```python
from build123d import *

# Parameters (mm, degrees)
CROQUIS1_R                 = 35
SALIENTE_EXTRUIR1_DEPTH    = 14
CROQUIS2_R                 = 17.5
CORTAR_EXTRUIR1_DEPTH      = 52.439284598
VACIADO1_T                 = -2
CHAFL_N1_SIZE              = 0.5
CHAFL_N1_SIZE2             = 1.866025404
CROQUIS5_R                 = 2.5
SALIENTE_EXTRUIR2_DEPTH    = 14
REDONDEO2_R                = 4
CORTAR_EXTRUIR2_DEPTH      = 51.931326337
CORTAR_EXTRUIR2_DEPTH_BACK = 51.931326337
CORTAR_EXTRUIR3_DEPTH      = 51.931326474
CORTAR_EXTRUIR3_DEPTH_BACK = 51.931326474


with BuildPart() as part:
    # Croquis1 → Saliente-Extruir1 (new body)
    with BuildSketch(Plane.XY):
        Circle(CROQUIS1_R)
    extrude(amount=SALIENTE_EXTRUIR1_DEPTH)

    # Croquis2 → Cortar-Extruir1 (cut, through all)
    with BuildSketch(Plane.XY.offset(14)):
        Circle(CROQUIS2_R)
    extrude(amount=-CORTAR_EXTRUIR1_DEPTH, mode=Mode.SUBTRACT)

    # Vaciado1
    vaciado1_openings = [part.faces().sort_by_distance(p)[0] for p in [
        (-34.010050506, 0, 14),
    ]]
    offset(amount=VACIADO1_T, openings=vaciado1_openings, kind=Kind.INTERSECTION)

    # Chaflán1
    chafl_n1_edges = [part.edges().sort_by_distance(p)[0] for p in [
        (-17.5, 0, 14),
    ]]
    chafl_n1_side = [part.faces().sort_by_distance(p)[0] for p in [
        (-18.948456711, 0, 14),
    ]]
    chamfer(chafl_n1_edges, length=CHAFL_N1_SIZE, length2=CHAFL_N1_SIZE2, reference=chafl_n1_side[0])

    # Croquis5 → Saliente-Extruir2 (add, through all)
    with BuildSketch(Plane(origin=(0, 0, 0), x_dir=(-1, 0, 0), z_dir=(0, 0, -1))):
        with Locations((0, 17.5)):
            Circle(CROQUIS5_R)
    extrude(amount=-SALIENTE_EXTRUIR2_DEPTH)

    # Redondeo1: read off the stored shape, not the designer's step
    # Redondeo1 outline → Redondeo1 (revolve)
    with BuildSketch(Plane.XZ):
        with BuildLine():
            ThreePointArc((21.5, 2), (20.085786438, 2.585786438), (19.5, 4))
            Line((19.5, 4), (19.5, 2))
            Line((19.5, 2), (21.5, 2))
        make_face()
        with BuildLine():
            ThreePointArc((33, 4), (32.414213562, 2.585786438), (31, 2))
            Line((31, 2), (33, 2))
            Line((33, 2), (33, 4))
        make_face()
    revolve(axis=Axis((0, 0, 0), (0, 0, 1)))

    # Redondeo2
    redondeo2_edges = [part.edges().sort_by_distance(p)[0] for p in [
        (-35, 0, 0),
    ]]
    fillet(redondeo2_edges, radius=REDONDEO2_R)

    # Croquis3 → Cortar-Extruir2 (cut, two sides: drawn at the far end of the back side and taken through both)
    with BuildSketch(Plane.XY.offset(2).offset(-CORTAR_EXTRUIR2_DEPTH_BACK)):
        with BuildLine():
            Line((8.410016673, 26.432172655), (2.046055643, 20.068211625))
            ThreePointArc((2.046055643, 20.068211625), (-2.196585045, 20.068211625), (-2.196585045, 24.310852312))
            Line((-2.196585045, 24.310852312), (4.167375986, 30.674813342))
            ThreePointArc((4.167375986, 30.674813342), (8.410016673, 30.674813342), (8.410016673, 26.432172655))
        make_face()
    extrude(amount=CORTAR_EXTRUIR2_DEPTH + CORTAR_EXTRUIR2_DEPTH_BACK, mode=Mode.SUBTRACT)

    # Croquis4 → Cortar-Extruir3 (cut, two sides: drawn at the far end of the back side and taken through both)
    with BuildSketch(Plane.XY.offset(2).offset(-CORTAR_EXTRUIR3_DEPTH_BACK)):
        Polygon((5.089600939, 21.651424089), (4.627973548, 20.226390042), (6.318861503, 19.678641589), (6.081885084, 18.947100367), (7.993733444, 19.923368498), (7.017465313, 21.835216858), (6.780488894, 21.103675636), align=None)
    extrude(amount=CORTAR_EXTRUIR3_DEPTH + CORTAR_EXTRUIR3_DEPTH_BACK, mode=Mode.SUBTRACT)


solid = part.part
```
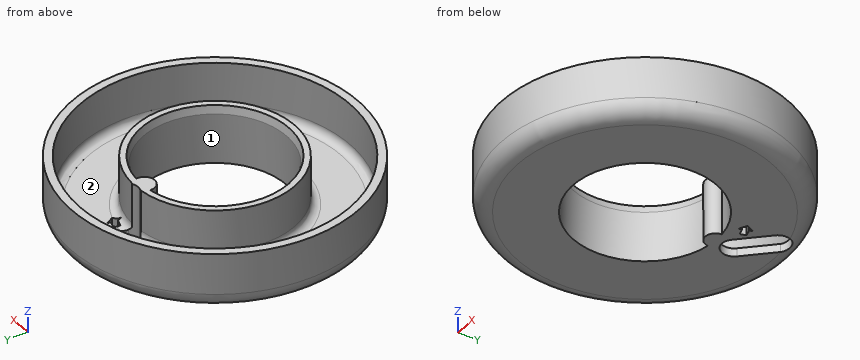
Verification items for the finished model (mm, model axes). Face numbers are marked on the shaded views. A direction names the side the tool comes from. Coordinates: 2 decimals unless noted, no trailing zeros. Loops run counter-clockwise (first coordinate to the right, second up) from the corner with the lowest first, then second, coordinate; pieces in that order, holes last. Notation, with made-up numbers: (46, 75.5) - (101, 75.5) arc R17 cw to (101, 81.5) - close; hole circle Ø4 at (77, 60). An arc over 180 degrees is marked (long way). Return JSON: item names as keys, results as strings.
1. Section check B-B, the plane z = 7.25. Record the boundary of the cut face in (x, y), then the cut area to 3 significant figures.
Established:
{"outline": "circle Ø70 at (0, 0); (-1.58, 19.44) arc R19.5 ccw (long way) to (1.58, 19.44) arc R2.5 ccw to (1.4, 19.57) arc R3 cw to (-1.46, 19.53) arc R2.5 ccw to start; hole circle Ø66 at (0, 0); hole (-2.49, 17.32) arc R17.5 ccw (long way) to (2.49, 17.32) arc R2.5 cw to start", "area": "669 mm2"}
2. Section check A-A, the plane y = 0. Record the boundary of the cut face in (x, z), then the cut area to 3 significant figures.
Established:
{"outline": "(-35, 4) arc R4 ccw to (-31, 0) - (-17.5, 0) - (-17.5, 12.13) - (-18, 14) - (-19.5, 14) - (-19.5, 4) arc R2 cw to (-21.5, 2) - (-31, 2) arc R2 cw to (-33, 4) - (-33, 14) - (-35, 14) - close; (17.5, 0) - (31, 0) arc R4 ccw to (35, 4) - (35, 14) - (33, 14) - (33, 4) arc R2 cw to (31, 2) - (21.5, 2) arc R2 cw to (19.5, 4) - (19.5, 14) - (18, 14) - (17.5, 12.13) - close", "area": "162 mm2"}
3. Tool access check on the marked faces 1 and 2. Record the directions out of +Z, -Z, +X, -X, +Y, -Y that give a thin tool (end or side, any length) a straight path to the whole face; none if there is none.
Established:
{"face 1": "+Z, -Z", "face 2": "+Z"}
4. Thickness scan on L1, parallel to Y at x = -1, z = 5.5; L2, parallel to X at y = -9.5, z = 5.5; L3, parallel to X at y = 11, z = 5.75. Record the ranges inside material, lowest first.
Established:
{"L1": "y = -34.99 to -32.98, -19.47 to -17.47, 15.21 to 19.34, 32.98 to 34.99", "L2": "x = -33.69 to -31.6, -17.03 to -14.7, 14.7 to 17.03, 31.6 to 33.69", "L3": "x = -33.23 to -31.11, -16.1 to -13.61, 13.61 to 16.1, 31.11 to 33.23"}
5. Section check C-C, the plane x = 0. Record the boundary of the cut face in (y, z), then the cut area to 3 significant figures.
Established:
{"outline": "(-35, 4) arc R4 ccw to (-31, 0) - (-17.5, 0) - (-17.5, 12.13) - (-18, 14) - (-19.5, 14) - (-19.5, 4) arc R2 cw to (-21.5, 2) - (-31, 2) arc R2 cw to (-33, 4) - (-33, 14) - (-35, 14) - close; (15, 0) - (19.19, 0) - (19.19, 14) - (15, 14) - close; (26.51, 0) - (31, 0) arc R4 ccw to (35, 4) - (35, 14) - (33, 14) - (33, 4) arc R2 cw to (31, 2) - (26.51, 2) - close", "area": "178 mm2"}
6. Go/stop test with flat-tipped pins: pin 1 (1 mm diameter, centred on x = 18, z = 8.5, fed in from +Y); pin 2 (2 mm diameter, centred on y = -3, z = 3.5, fed in from -X); pin 3 (1.5 mm diameter, centred on y = -15.5, z = 2.5, fed in from +X). Record where each tip stops, or that it passes through.
Established:
{"pin 1": "stops at y = 30.31", "pin 2": "stops at x = -34.94", "pin 3": "stops at x = 31.52"}
